The listing builds one solid part. Answer for the finished solid, in the listing's coordinates (mm). A direction names the side the tool comes from. Coordinates: 2 decimals unless noted, no trailing zeros. Write each loop counter-clockwise with the first axis right and the second up, starting at its lowest first coordinate (ties: lowest second). Pieces come first, ordered by that corner, then holes.
Autodesk Inventor part; units mm, degrees
ref_plane "YZ Plane" through (0, 0, 0) normal (1, 0, 0) x (0, 1, 0)
ref_plane "XZ Plane" through (0, 0, 0) normal (0, 1, 0) x (-1, 0, 0)
ref_plane "XY Plane" through (0, 0, 0) normal (0, 0, 1) x (1, 0, 0)
sketch "スケッチ1" plane through (0, 0, 0) normal (0, 0, 1) x (1, 0, 0)
  point P0 (0, 0)
sketch "スケッチ2" plane through (0, 0, 0) normal (0, 1, 0) x (-1, 0, 0)
  line L0 (7.625, 9.25) -> (-7.625, 9.25)
  line L1 (-9.625, 7.25) -> (-9.625, -7.25)
  line L2 (-7.625, -9.25) -> (7.625, -9.25)
  line L3 (9.625, -7.25) -> (9.625, 7.25)
  line L4 (9.625, 9.25) -> (-9.625, -9.25) construction
  line L5 (-9.625, 9.25) -> (9.625, -9.25) construction
  circle A0 centre (7.625, -7.25) radius 1.05
  arc A1 (7.625, -9.25) -> (9.625, -7.25) centre (7.625, -7.25) ccw
  circle A2 centre (7.625, 7.25) radius 1.05
  arc A3 (9.625, 7.25) -> (7.625, 9.25) centre (7.625, 7.25) ccw
  circle A4 centre (-7.625, 7.25) radius 1.05
  circle A5 centre (-7.625, -7.25) radius 1.05
  arc A6 (-7.625, 9.25) -> (-9.625, 7.25) centre (-7.625, 7.25) ccw
  arc A7 (-9.625, -7.25) -> (-7.625, -9.25) centre (-7.625, -7.25) ccw
  point P0 (0, 0)
  dimension "d0" = 19.25
  dimension "d1" = 18.5
  dimension "ねじ穴" = 2.1
  dimension "d6" = 2
  dimension "d7" = 2
  dimension "d8" = 2
  dimension "d9" = 2
  dimension "d10" = 2.1
  dimension "d11" = 2.1
  dimension "d12" = 2.1
  dimension "d13" = 2
  dimension "d14" = 2
  dimension "d15" = 2
  dimension "d16" = 2
extrude "押し出し1" add sketch "スケッチ2" along normal blind 5
sketch "スケッチ3" plane through (9.625, 0, 7.25) normal (1, 0, 0) x (0, 0, -1)
  line L0 (0, 5) -> (14.5, 5)
  circle A0 centre (7.25, 5) radius 3.25
  point P0 (7.25, 0)
  dimension "d19" = 6.5
extrude "押し出し2" cut sketch "スケッチ3" against normal blind 17.5
sketch "スケッチ4" plane through (0, 0, 0) normal (0, -1, 0) x (1, 0, 0)
  circle A0 centre (-7.625, 7.25) radius 1.05
  circle A1 centre (-7.625, 7.25) radius 2.25
  circle A2 centre (7.625, 7.25) radius 1.05
  circle A3 centre (7.625, 7.25) radius 2.25
  circle A4 centre (7.625, -7.25) radius 1.05
  circle A5 centre (7.625, -7.25) radius 2.25
  circle A6 centre (-7.625, -7.25) radius 1.05
  circle A7 centre (-7.625, -7.25) radius 2.25
  point P0 (0, 0)
  dimension "d22" = 4.5
  dimension "d23" = 4.5
  dimension "d24" = 4.5
  dimension "d25" = 4.5
extrude "押し出し3" cut sketch "スケッチ4" against normal blind 2
fillet "フィレット1" radius 2 4 edges at (0, 0, 9.25) (-9.625, 0, 0) (0, 0, -9.25) (9.625, 0, 0)
sketch "スケッチ5" plane through (0, 0, 0) normal (0, -1, 0) x (1, 0, 0)
  line L0 (-0.875, 3.4) -> (7.625, 3.4)
  line L1 (7.625, 3.4) -> (7.625, -3.4)
  line L2 (7.625, -3.4) -> (-0.875, -3.4)
  line L3 (-0.875, -3.4) -> (-0.875, 3.4)
  line L4 (9.625, 1.25) -> (9.625, 6.2192)
  point P0 (0, 0)
  point P1 (-0.875, 0)
  dimension "d29" = 2
  dimension "d30" = 6.8
  dimension "d31" = 8.5
  dimension "d32" = 0
extrude "押し出し4" cut sketch "スケッチ5" against normal through all
sketch "スケッチ6" plane through (0, 5, 0) normal (0, 1, 0) x (1, 0, 0)
  line L0 (7.625, -5.4) -> (-0.875, -5.4)
  line L1 (-0.875, -5.4) -> (-0.875, 5.4)
  line L2 (-0.875, 5.4) -> (7.625, 5.4)
  line L3 (7.625, 5.4) -> (7.625, -5.4)
  line L4 (9.625, -7.25) -> (9.625, -3.25)
  point P0 (0, 0)
  point P1 (-0.875, 0)
  point P2 (-0.875, -3.4)
  point P3 (7.625, -3.4)
  dimension "d35" = 2
  dimension "d36" = 8.5
  dimension "d37" = 10.8
  dimension "d38" = 0
  dimension "d39" = 8.5
extrude "押し出し5" cut sketch "スケッチ6" against normal blind 1.25
equation "\"d7\" = d6"
equation "\"d8\" = d6"
equation "\"d9\" = d6"
equation "\"d10\" = ねじ穴"
equation "\"d11\" = ねじ穴"
equation "\"d12\" = ねじ穴"
equation "\"d13\" = d6"
equation "\"d14\" = d6"
equation "\"d15\" = d6"
equation "\"d16\" = d6"
equation "\"d23\" = d22"
equation "\"d24\" = d22"
equation "\"d25\" = d22"
equation "\"d36\" = d39"
properties part number "カバー"
Q1. Find the intervals of material crossed by probe 1 along X at (y, z) = (4.05, -7.25) (3 decimals); probe 2 along X at (y, z) = (2.65, -8); probe 3 along Z at (x, y) = (2.5, 4.2), in increasing order.
Answers below:
probe 1: x = -9.625 to -8.675, -6.575 to 6.575, 8.675 to 9.625
probe 2: x = -9.48 to -8.36, -6.89 to 6.89, 8.36 to 9.48
probe 3: z = -9.25 to -5.4, 5.4 to 9.25
Q2. Which of the six approach directions +Z, -Z, +X, -X, +Y, -Y give full straight-line access (tool end or side, diameter ignored) to faces 1 (the face through (8.64, 1.75, 0.07)), 2 (the face through (-7, 2, 6)), 3 (the face through (-8.189, 3.479, -8.135)), 4 (the face through (-9.055, 0.601, 0.087)), 5 (the face through (3, 4, -5.4))?
Answers below:
face 1: +X, +Y
face 2: -Y
face 3: +Y, -Y
face 4: +Z, -Z, -X, -Y
face 5: +Y
Q3. The part is cut by section A-A, the plane y = 2.7. Write down the section's boundary in (x, z) (3 decimals), then the cut area to 3 significant figures.
Answers below:
outline: (-9.625, -7.25) arc R2 ccw to (-7.625, -9.25) - (7.625, -9.25) arc R2 ccw to (9.625, -7.25) - (9.625, -2.296) - (7.625, -2.296) - (7.625, -3.4) - (-0.875, -3.4) - (-0.875, -2.296) - (-7.875, -2.296) - (-7.875, 2.296) - (-0.875, 2.296) - (-0.875, 3.4) - (7.625, 3.4) - (7.625, 2.296) - (9.625, 2.296) - (9.625, 7.25) arc R2 ccw to (7.625, 9.25) - (-7.625, 9.25) arc R2 ccw to (-9.625, 7.25) - close; hole circle Ø2.1 at (-7.625, -7.25); hole circle Ø2.1 at (-7.625, 7.25); hole circle Ø2.1 at (7.625, -7.25); hole circle Ø2.1 at (7.625, 7.25)
area: 240 mm2
Q4. Given pin 1 (1.6 mm diameter, centred on x = 2, z = -4.5, fed in from +Y); pin 2 (4 mm diameter, centred on x = 7.625, z = -7.25, fed in from -Y), each flat-ended and moving along its own axis, determine where each tip first touches the part or whether it passes through.
Answers below:
pin 1: stops at y = 3.75
pin 2: stops at y = 2
Q5. The part is cut by section C-C, the plane z = 4. Write down the section's boundary in (x, y) (3 decimals), then the cut area to 3 significant figures.
Answers below:
outline: (-9.625, 2) arc R2 ccw to (-7.625, 0) - (7.625, 0) arc R2 ccw to (9.625, 2) - (9.625, 5) - (7.625, 5) - (7.625, 3.75) - (-0.875, 3.75) - (-0.875, 5) - (-9.625, 5) - close
area: 83.9 mm2
Q6. The part is cut by section D-D, the plane y = 4.2. Write down the section's boundary in (x, z) (3 decimals).
Answers below:
outline: (-9.625, -7.25) arc R2 ccw to (-7.625, -9.25) - (7.625, -9.25) arc R2 ccw to (9.625, -7.25) - (9.625, -3.15) - (7.625, -3.15) - (7.625, -5.4) - (-0.875, -5.4) - (-0.875, -3.15) - (-7.875, -3.15) - (-7.875, 3.15) - (-0.875, 3.15) - (-0.875, 5.4) - (7.625, 5.4) - (7.625, 3.15) - (9.625, 3.15) - (9.625, 7.25) arc R2 ccw to (7.625, 9.25) - (-7.625, 9.25) arc R2 ccw to (-9.625, 7.25) - close; hole circle Ø2.1 at (-7.625, -7.25); hole circle Ø2.1 at (-7.625, 7.25); hole circle Ø2.1 at (7.625, -7.25); hole circle Ø2.1 at (7.625, 7.25)
Q7. The part is cut by section B-B, the plane z = 7.75. Write down the section's boundary in (x, y).
Answers below:
outline: (-9.56, 2) - (-8.55, 2) - (-8.55, 5) - (-9.56, 5) - close; (-6.7, 2) - (-5.43, 2) - (-5.43, 0.06) - (5.43, 0.06) - (5.43, 2) - (6.7, 2) - (6.7, 5) - (-6.7, 5) - close; (8.55, 2) - (9.56, 2) - (9.56, 5) - (8.55, 5) - close
